from build123d import *

# Parameters (mm, degrees)
SKETCH1_W           = 45.4
SKETCH1_H           = 50
BOSS_EXTRUDE1_DEPTH = 15.5
SKETCH2_W           = 45.4
SKETCH2_H           = 27
CUT_EXTRUDE1_DEPTH  = 8
SKETCH7_W           = 45.4
SKETCH7_H           = 5
BOSS_EXTRUDE2_DEPTH = 18
SKETCH8_W           = 45.4
SKETCH8_H           = 12
BOSS_EXTRUDE3_DEPTH = 12.52
CUT_EXTRUDE2_REACH  = 77.388
SKETCH11_W          = 7
SKETCH11_H          = 2.6
CUT_EXTRUDE3_DEPTH  = 70.893919621
FILLET1_SIZE        = 2.5
FILLET1_SIZE_2      = 8
CUT_EXTRUDE4_REACH  = 77.388
SKETCH13_R          = 1.7
SKETCH14_W          = 8
SKETCH14_H          = 1.5
BOSS_EXTRUDE4_DEPTH = 11
FILLET3_R           = 10
FILLET4_R           = 10
SKETCH15_R          = 1.7
CUT_EXTRUDE6_DEPTH  = 81.878983729
SKETCH16_R          = 3.5
CUT_EXTRUDE7_DEPTH  = 80.267963321
SKETCH17_R          = 4
CUT_EXTRUDE8_DEPTH  = 2.2
FILLET5_R           = 5
FILLET6_R           = 5
FILLET7_R           = 5
SKETCH18_R          = 1.35
CUT_EXTRUDE9_DEPTH  = 10


with BuildPart() as part:
    # Sketch1 → Boss-Extrude1 (new body)
    with BuildSketch(Plane.XY):
        with Locations((22.7, 25)):
            Rectangle(SKETCH1_W, SKETCH1_H)
    extrude(amount=BOSS_EXTRUDE1_DEPTH)

    # Sketch2 → Cut-Extrude1 (cut)
    with BuildSketch(Plane(origin=(0, 0, 0), x_dir=(-1, 0, 0), z_dir=(0, 0, -1))):
        with Locations((-22.7, 23.263256753)):
            Rectangle(SKETCH2_W, SKETCH2_H)
    extrude(amount=-CUT_EXTRUDE1_DEPTH, mode=Mode.SUBTRACT)

    # Sketch7 → Boss-Extrude2 (add)
    with BuildSketch(Plane(origin=(0, 0, 0), x_dir=(-1, 0, 0), z_dir=(0, 0, -1))):
        with Locations((-22.7, 39.263256753)):
            Rectangle(SKETCH7_W, SKETCH7_H)
    extrude(amount=BOSS_EXTRUDE2_DEPTH)

    # Sketch8 → Boss-Extrude3 (add)
    with BuildSketch(Plane.XZ.offset(-36.763256753)):
        with Locations((22.7, -12)):
            Rectangle(SKETCH8_W, SKETCH8_H)
    extrude(amount=BOSS_EXTRUDE3_DEPTH)

    # Sketch10 → Cut-Extrude2 (cut, up to next)
    with BuildSketch(Plane(origin=(0, 0, -18), x_dir=(-1, 0, 0), z_dir=(0, 0, -1)), mode=Mode.PRIVATE) as cut_extrude2_sk1:
        with BuildLine():
            Line((-37, 27.243256753), (-8, 27.243256753))
            ThreePointArc((-8, 27.243256753), (-9.5, 25.743256753), (-8, 24.243256753))
            Line((-8, 24.243256753), (-37, 24.243256753))
            ThreePointArc((-37, 24.243256753), (-35.5, 25.743256753), (-37, 27.243256753))
        make_face()
    cut_extrude2_tool1 = extrude(cut_extrude2_sk1.sketch, amount=-CUT_EXTRUDE2_REACH, mode=Mode.PRIVATE) & part.part
    add(cut_extrude2_tool1.solids().sort_by_distance((22.5, 25.743257, -18))[0], mode=Mode.SUBTRACT)

    # Sketch11 → Cut-Extrude3 (cut, through all)
    with BuildSketch(Plane(origin=(45.4, 0, 0), x_dir=(0, 0, -1), z_dir=(1, 0, 0))):
        with Locations((12, 28.543256753)):
            Rectangle(SKETCH11_W, SKETCH11_H)
    extrude(amount=-CUT_EXTRUDE3_DEPTH, mode=Mode.SUBTRACT)

    # Fillet1
    # an asymmetric fillet: 8, 2.5 mm, written as the material it takes off along each edge
    with BuildSketch(Plane(origin=(0, 24.243256753, 14), x_dir=(0, 1, 0), z_dir=(0, 0, -1))) as fillet1_piece_1_section:
        with BuildLine():
            Bezier((FILLET1_SIZE, 0), (0, 0), (0, FILLET1_SIZE_2), weights=[1, 0.707106781, 1])
            Line((0, FILLET1_SIZE_2), (0, 0))
            Line((0, 0), (FILLET1_SIZE, 0))
        make_face()
    fillet1_piece_1 = extrude(amount=52, mode=Mode.PRIVATE)
    fillet1_piece_1 = split(fillet1_piece_1, bisect_by=Plane(origin=(1.786931274, 24.8016736, 8), z_dir=(0, 0, -1)), keep=Keep.TOP, mode=Mode.PRIVATE)
    add(fillet1_piece_1, mode=Mode.SUBTRACT)
    with BuildSketch(Plane(origin=(45.4, 24.243256753, -38), x_dir=(0, 1, 0), z_dir=(0, 0, 1))) as fillet1_piece_2_section:
        with BuildLine():
            Bezier((FILLET1_SIZE, 0), (0, 0), (0, FILLET1_SIZE_2), weights=[1, 0.707106781, 1])
            Line((0, FILLET1_SIZE_2), (0, 0))
            Line((0, 0), (FILLET1_SIZE, 0))
        make_face()
    fillet1_piece_2 = extrude(amount=52, mode=Mode.PRIVATE)
    fillet1_piece_2 = split(fillet1_piece_2, bisect_by=Plane(origin=(43.613068726, 24.8016736, 8), z_dir=(0, 0, -1)), keep=Keep.TOP, mode=Mode.PRIVATE)
    add(fillet1_piece_2, mode=Mode.SUBTRACT)

    # Sketch13 → Cut-Extrude4 (cut, up to next)
    with BuildSketch(Plane.XY.offset(15.5), mode=Mode.PRIVATE) as cut_extrude4_sk1:
        with Locations((12.7, 33.263245951)):
            Circle(SKETCH13_R)
    cut_extrude4_tool1 = extrude(cut_extrude4_sk1.sketch, amount=-CUT_EXTRUDE4_REACH, mode=Mode.PRIVATE) & part.part
    # Sketch13 → Cut-Extrude4 (cut, up to next)
    with BuildSketch(Plane.XY.offset(15.5), mode=Mode.PRIVATE) as cut_extrude4_sk2:
        with Locations((32.7, 33.263245951)):
            Circle(SKETCH13_R)
    cut_extrude4_tool2 = extrude(cut_extrude4_sk2.sketch, amount=-CUT_EXTRUDE4_REACH, mode=Mode.PRIVATE) & part.part
    # Sketch13 → Cut-Extrude4 (cut, up to next)
    with BuildSketch(Plane.XY.offset(15.5), mode=Mode.PRIVATE) as cut_extrude4_sk3:
        with Locations((32.7, 13.263245951)):
            Circle(SKETCH13_R)
    cut_extrude4_tool3 = extrude(cut_extrude4_sk3.sketch, amount=-CUT_EXTRUDE4_REACH, mode=Mode.PRIVATE) & part.part
    # Sketch13 → Cut-Extrude4 (cut, up to next)
    with BuildSketch(Plane.XY.offset(15.5), mode=Mode.PRIVATE) as cut_extrude4_sk4:
        with Locations((12.7, 13.263245951)):
            Circle(SKETCH13_R)
    cut_extrude4_tool4 = extrude(cut_extrude4_sk4.sketch, amount=-CUT_EXTRUDE4_REACH, mode=Mode.PRIVATE) & part.part
    add(cut_extrude4_tool1.solids().sort_by_distance((12.7, 33.263246, 15.5))[0], mode=Mode.SUBTRACT)
    add(cut_extrude4_tool2.solids().sort_by_distance((32.7, 33.263246, 15.5))[0], mode=Mode.SUBTRACT)
    add(cut_extrude4_tool3.solids().sort_by_distance((32.7, 13.263246, 15.5))[0], mode=Mode.SUBTRACT)
    add(cut_extrude4_tool4.solids().sort_by_distance((12.7, 13.263246, 15.5))[0], mode=Mode.SUBTRACT)

    # Sketch14 → Boss-Extrude4 (add)
    with BuildSketch(Plane(origin=(0, 0, -18), x_dir=(-1, 0, 0), z_dir=(0, 0, -1))):
        with Locations((-4, 27.993256753)):
            Rectangle(SKETCH14_W, SKETCH14_H)
    extrude(amount=BOSS_EXTRUDE4_DEPTH)

    # Fillet3
    # the kernel refuses this fillet: 10 mm, written as the material it adds along each edge
    with BuildSketch(Plane(origin=(8, 28.743256753, -18), x_dir=(1, 0, 0), z_dir=(0, -1, 0))) as fillet3_piece_1:
        with BuildLine():
            CenterArc((FILLET3_R, -FILLET3_R), FILLET3_R, 90, 90)
            Line((0, -FILLET3_R), (0, 0))
            Line((0, 0), (FILLET3_R, 0))
        make_face()
    extrude(amount=1.5)

    # Fillet4
    # the kernel refuses this fillet: 10 mm, written as the material it takes off along each edge
    with BuildSketch(Plane(origin=(8, 48.394684502, -29), x_dir=(-1, 0, 0), z_dir=(0, -1, 0))) as fillet4_piece_1:
        with BuildLine():
            CenterArc((7.860571099, -10), FILLET4_R, 90, 63.25631605)
            Line((-1.06971445, -5.5), (-1.962743005, -5.05))
            ThreePointArc((-1.962743005, -5.05), (-1, -1), (-1, 0))
            Line((-1, 0), (0, 1))
            Line((0, 1), (7.860571099, 1))
            Line((7.860571099, 1), (7.860571099, 0))
        make_face()
    extrude(amount=40.802855497, mode=Mode.SUBTRACT)

    # Sketch15 → Cut-Extrude6 (cut, through all)
    with BuildSketch(Plane(origin=(0, 0, 15.5), x_dir=(-1, 0, 0), z_dir=(0, 0, -1))):
        with Locations((-5.2, 45)):
            Circle(SKETCH15_R)
        with Locations((-40.2, 45)):
            Circle(SKETCH15_R)
        with Locations((-40.2, 5)):
            Circle(SKETCH15_R)
        with Locations((-5.2, 5)):
            Circle(SKETCH15_R)
    extrude(amount=CUT_EXTRUDE6_DEPTH, mode=Mode.SUBTRACT)

    # Sketch16 → Cut-Extrude7 (cut, through all)
    with BuildSketch(Plane.XY.offset(12.5)):
        with Locations((5.2, 45)):
            Circle(SKETCH16_R)
        with Locations((40.2, 45)):
            Circle(SKETCH16_R)
        with Locations((40.2, 5)):
            Circle(SKETCH16_R)
        with Locations((5.2, 5)):
            Circle(SKETCH16_R)
    extrude(amount=-CUT_EXTRUDE7_DEPTH, mode=Mode.SUBTRACT)

    # Sketch17 → Cut-Extrude8 (cut)
    with BuildSketch(Plane.XY.offset(15.5)):
        with Locations((12.7, 33.263245951)):
            Circle(SKETCH17_R)
        with Locations((32.7, 33.263245951)):
            Circle(SKETCH17_R)
        with Locations((32.7, 13.263245951)):
            Circle(SKETCH17_R)
        with Locations((12.7, 13.263245951)):
            Circle(SKETCH17_R)
    extrude(amount=-CUT_EXTRUDE8_DEPTH, mode=Mode.SUBTRACT)

    # Fillet5
    fillet5_edges = [part.edges().sort_by_distance(p)[0] for p in [
        (22.7, 36.763256753, -6),
    ]]
    fillet(fillet5_edges, radius=FILLET5_R)

    # Fillet6
    fillet6_edges = [part.edges().sort_by_distance(p)[0] for p in [
        (22.7, 41.763256753, -18),
    ]]
    fillet(fillet6_edges, radius=FILLET6_R)

    # Fillet7
    # the kernel refuses this fillet: 5 mm, written as the material it adds along each edge
    with BuildSketch(Plane(origin=(51.368274369, 41.763256753, 0), x_dir=(0, 1, 0), z_dir=(-1, 0, 0))) as fillet7_piece_1_section:
        with BuildLine():
            CenterArc((FILLET7_R, FILLET7_R), FILLET7_R, 180, 90)
            Line((0, FILLET7_R), (0, 0))
            Line((0, 0), (FILLET7_R, 0))
        make_face()
    fillet7_piece_1 = extrude(amount=57.336548738, mode=Mode.PRIVATE)
    fillet7_piece_1 = split(fillet7_piece_1, bisect_by=Plane(origin=(0, 42.669837738, -1.260146255), z_dir=(1, 0, 0)), keep=Keep.TOP, mode=Mode.PRIVATE)
    fillet7_piece_1 = split(fillet7_piece_1, bisect_by=Plane(origin=(45.4, 42.669837738, -1.260146255), z_dir=(-1, 0, 0)), keep=Keep.TOP, mode=Mode.PRIVATE)
    fillet7_piece_1 = fillet7_piece_1 - Plane(origin=(40.2, 45, -1.260146255), x_dir=(1, 0, 0), z_dir=(0, 0, 1)) * Cylinder(3.5, 135, mode=Mode.PRIVATE)
    fillet7_piece_1 = fillet7_piece_1 - Plane(origin=(5.2, 45, -1.260146255), x_dir=(1, 0, 0), z_dir=(0, 0, 1)) * Cylinder(3.5, 135, mode=Mode.PRIVATE)
    with BuildSketch(Plane(origin=(45.4, 41.763256753, 0), x_dir=(0, 1, 0), z_dir=(-1, 0, 0))) as fillet7_piece_2_section:
        with BuildLine():
            CenterArc((FILLET7_R, FILLET7_R), FILLET7_R, 180, 90)
            Line((0, FILLET7_R), (0, 0))
            Line((0, 0), (FILLET7_R, 0))
        make_face()
    fillet7_piece_2 = extrude(amount=16.368274369, mode=Mode.PRIVATE)
    fillet7_piece_2 = fillet7_piece_2 - Plane(origin=(40.2, 45, -1.260146255), x_dir=(1, 0, 0), z_dir=(0, 0, 1)) * Cylinder(3.5, 53, mode=Mode.PRIVATE)
    with BuildSketch(Plane(origin=(16.368274369, 41.763256753, 0), x_dir=(0, 0, -1), z_dir=(-1, 0, 0))) as fillet7_piece_3_section:
        with BuildLine():
            CenterArc((FILLET7_R, -FILLET7_R), FILLET7_R, 90, 90)
            Line((0, -FILLET7_R), (0, 0))
            Line((0, 0), (FILLET7_R, 0))
        make_face()
    fillet7_piece_3 = extrude(amount=16.368274369, mode=Mode.PRIVATE)
    fillet7_piece_3 = fillet7_piece_3 - Plane(origin=(5.2, 45, -1.161012309), x_dir=(1, 0, 0), z_dir=(0, 0, 1)) * Cylinder(3.5, 53, mode=Mode.PRIVATE)
    add([fillet7_piece_1, fillet7_piece_2, fillet7_piece_3])

    # Sketch18 → Cut-Extrude9 (cut)
    with BuildSketch(Plane(origin=(0, 0, 0), x_dir=(-1, 0, 0), z_dir=(0, 0, -1))):
        with Locations((-32.4, 4.881628377)):
            Circle(SKETCH18_R)
        with Locations((-13, 4.881628377)):
            Circle(SKETCH18_R)
    extrude(amount=-CUT_EXTRUDE9_DEPTH, mode=Mode.SUBTRACT)


solid = part.part
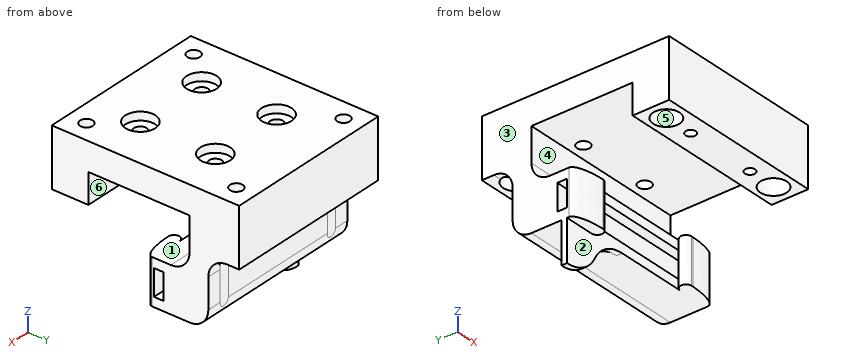
Geometry check sheet. Reference: the model listing, model coordinates, mm. Face numbers are marked on the shaded views. A direction names the side the tool comes from. Give positions to 0.01 mm unless a question says otherwise; leave off trailing zeros. Write each loop counter-clockwise with the first axis right and the second up, starting at its lowest first coordinate (ties: lowest second). Pieces come first, ordered by that corner, then holes.
1) Thickness scan on line 1 (Y direction, x = 5.2, z = 14); line 2 (Z direction, x = 20.5, y = 29); line 3 (Y direction, x = 12.7, z = 11). Record the ranges inside material, lowest first.
Values follow:
line 1: y = 0 to 3.3, 6.7 to 43.3, 46.7 to 50
line 2: z = -18 to -15.5, -8.5 to -6, 8 to 15.5
line 3: y = 0 to 11.56, 14.96 to 31.56, 34.96 to 50
2) Go/stop test with flat-tipped pins: pin 1 Ø4 at (x, z) = (15, -15.5) entering from +Y; pin 2 Ø4 at (x, z) = (38, -16.5) entering from -Y; pin 3 Ø4 at (x, y) = (5.2, 45) entering from -Z. Record where each tip stops, or that it passes through.
Values follow:
pin 1: stops at y = 41.74
pin 2: stops at y = 24.24
pin 3: stops at z = 12.5
3) Release check for a two-part mould opening along X. For the marked faces 1, 2 and 3 record: released by +X, released by -X, zero draft, split by the parting line, or undercut.
Values follow:
face 1: zero draft
face 2: undercut
face 3: released by -X
4) Cross-section at D-D (y = 19). Record the boundary of the cut face in (x, z), plus the area to 4 significant figures.
Values follow:
outline: (0, 8) - (45.4, 8) - (45.4, 15.5) - (0, 15.5) - close
area: 340.5 mm2
5) Cross-section at B-B (z = -9.5). Count the separate pieces of the cut face and the enclosed holes in it, plus the area to 3 significant figures.
Values follow:
separate pieces: 3
enclosed holes: 0
area: 588 mm2
6) Cross-section at A-A (z = 7). Record the boundary of the cut face in (x, y).
Values follow:
outline: (0, 0) - (45.4, 0) - (45.4, 9.76) - (0, 9.76) - close; (0, 36.76) - (45.4, 36.76) - (45.4, 50) - (0, 50) - close; hole circle Ø7 at (5.2, 5); hole circle Ø7 at (5.2, 45); hole circle Ø2.7 at (13, 4.88); hole circle Ø2.7 at (32.4, 4.88); hole circle Ø7 at (40.2, 5); hole circle Ø7 at (40.2, 45)
7) Set-up check for the marked faces 4, 5 and 6: record each of +Z, -Z, +X, -X, +Y, -Y from which the full face is reachable in a straight line by a thin tool's end or side.
Values follow:
face 4: +X, -X
face 5: -Z
face 6: -Z, +X, -X
